Autodesk Inventor part; units mm, degrees
ref_plane "YZ Plane" through (0, 0, 0) normal (1, 0, 0) x (0, 1, 0)
ref_plane "XZ Plane" through (0, 0, 0) normal (0, 1, 0) x (-1, 0, 0)
ref_plane "XY Plane" through (0, 0, 0) normal (0, 0, 1) x (1, 0, 0)
sketch "Sketch1" plane through (0, 0, 0) normal (0, 1, 0) x (-1, 0, 0)
  line L0 (0, 0) -> (-5, 0)
  line L1 (-5, 0) -> (-5, -120)
  line L2 (-5, -120) -> (0, -120)
  line L3 (0, -120) -> (0, 0)
  dimension "d0" = 5
  dimension "d1" = 120
extrude "Extrusion1" add sketch "Sketch1" along normal blind 100
sketch "Sketch2" plane through (0, 0, 0) normal (0, -1, 0) x (1, 0, 0)
  line L0 (0, -120) -> (0, 0)
  line L1 (0, 0) -> (2.5, 0)
  line L2 (2.5, 0) -> (2.5, -15)
  line L3 (2.5, -15) -> (0, -15)
  line L4 (0, -15) -> (0, 0)
  circle A0 centre (2.5, -15) radius 1.75
  dimension "d4" = 2.5
  dimension "d5" = 15
  dimension "d6" = 3.5
extrude "Extrusion2" add sketch "Sketch2" along normal blind 5 contours A0 L2 L3 | L3 L2 A0
sketch "Sketch3" plane through (0, 0, 0) normal (0, -1, 0) x (1, 0, 0)
  line L0 (5, 0) -> (5, -120)
  line L1 (5, -120) -> (2.5, -120)
  line L2 (2.5, -120) -> (2.5, -105)
  line L3 (2.5, -105) -> (5, -105)
  line L4 (5, -105) -> (5, -120)
  circle A0 centre (2.5, -105) radius 1.75
  point P0 (0, 0)
  dimension "d9" = 2.5
  dimension "d10" = 15
  dimension "d11" = 3.5
extrude "Extrusion3" add sketch "Sketch3" along normal blind 5 contours A0 L2 L3 | L3 L2 A0
sketch "Sketch4" plane through (5, 0, 0) normal (1, 0, 0) x (0, 0, -1)
  point P0 (0, 0)
sketch "Sketch5" plane through (5, 0, 0) normal (1, 0, 0) x (0, 0, -1)
  point P0 (0, 0)
sketch "Sketch6" plane through (5, 0, 0) normal (1, 0, 0) x (0, 0, -1)
  point P0 (0, 0)
sketch "Sketch7" plane through (5, 0, 0) normal (1, 0, 0) x (0, 0, -1)
  line L0 (120, 100) -> (0, 100)
  line L1 (0, 100) -> (42.838, 100)
  line L2 (42.838, 100) -> (42.838, 80)
  line L3 (42.838, 80) -> (0, 80)
  line L4 (0, 80) -> (0, 100)
  line L5 (42.838, 80) -> (77.174, 80)
  line L6 (77.174, 80) -> (77.174, 72)
  line L7 (77.174, 72) -> (42.838, 72)
  line L8 (42.838, 72) -> (42.838, 80)
  point P0 (0, 0)
  dimension "d14" = 42.838
  dimension "d15" = 20
  dimension "d16" = 34.336
  dimension "d17" = 8
extrude "Extrusion4" cut sketch "Sketch7" against normal blind 10 contours L5 L6 L7 L8
sketch "Sketch8" plane through (5, 0, 0) normal (1, 0, 0) x (0, 0, -1)
  line L0 (0, 0) -> (60, 0)
  line L1 (60, 0) -> (60, 15)
  line L2 (60, 15) -> (0, 15)
  line L3 (0, 15) -> (0, 0)
  line L4 (60, 15) -> (70, 15)
  line L5 (70, 15) -> (70, 20)
  line L6 (70, 20) -> (60, 20)
  line L7 (60, 20) -> (60, 15)
  dimension "d20" = 60
  dimension "d21" = 15
  dimension "d22" = 10
  dimension "d23" = 5
extrude "Extrusion5" cut sketch "Sketch8" against normal blind 10 contours L7 L6 L5 L4
properties part number "expo3"
Part model, mm, in its own coordinate system. A direction names the side the tool comes from. Give positions to 0.01 mm unless a question says otherwise; leave off trailing zeros. Order: outer loops, then holes, each group sorted by start corner. A loop starts at its lowest first (then second) coordinate and runs counter-clockwise, first axis right, second up. Notation, with made-up numbers: (58.25, -29.5) - (102.25, -29.5) arc R15 ccw to (102.25, -22.5) - close; hole circle Ø1 at (66.5, -1.5). An arc over 180 degrees is marked (long way). Use one line per item in the form item = value.
Item 1: Slice it at B-B on x = 2.5. Give the cut face in (y, z).
Solution:
outline = (-5, -106.75) - (0, -106.75) - (0, -120) - (100, -120) - (100, 0) - (0, 0) - (0, -13.25) - (-5, -13.25) - (-5, -16.75) - (0, -16.75) - (0, -103.25) - (-5, -103.25) - close; hole (15, -70) - (20, -70) - (20, -60) - (15, -60) - close; hole (72, -77.17) - (80, -77.17) - (80, -42.84) - (72, -42.84) - close
Item 2: Probe probe 1 along Z at (x, y) = (1.55, 19); probe 2 along Y at (x, z) = (2.05, -51); probe 3 along Y at (x, z) = (2.4, -24). List the from-to ranges inside material, lowest first. Write a range as from..to.
Solution:
probe_1 = -120..-70, -60..0
probe_2 = 0..72, 80..100
probe_3 = 0..100
Item 3: Slice it at C-C on z = -26.5. Give the cut face in (x, y).
Solution:
outline = (0, 0) - (5, 0) - (5, 100) - (0, 100) - close
Item 4: Two-plate mould, pull along Y, no slides. Class faces 4 (the face through (3, 18, -60)), 5 (the face through (3, 100, -59)), 6 (the face through (3, 17, -70)), 7 (the face through (2, -5, -105)): released by +Y, released by -Y, zero draft, split by the parting line, or undercut.
Solution:
face_4 = undercut
face_5 = released by +Y
face_6 = undercut
face_7 = released by -Y
Item 5: Which spindle directions (+Z, -Z, +X, -X, +Y, -Y) get a long thin tool onto all of the face, cutting with end or side? Do faces 1 (the face through (2.272, -2.465, -16.735)), 2 (the face through (3, 49, -120)), 3 (the face through (3, 76, -77.174)). Say none if no direction does.
Solution:
face_1 = -Y
face_2 = -Z, +X, -X, +Y, -Y
face_3 = +X, -X
Item 6: Slice it at A-A on y = 77.5. Give the cut face in (x, z).
Solution:
outline = (0, -120) - (5, -120) - (5, -77.17) - (0, -77.17) - close; (0, -42.84) - (5, -42.84) - (5, 0) - (0, 0) - close
Item 7: Pin check, flat tip, straight feed: pin 1 Ø3 at (x, z) = (2, -22) entering from -Y. Stop position of the tip, or through.
Solution:
pin_1 = 0
